from build123d import *

# Parameters (mm, degrees)
SKETCH1_R               = 19.53
BOSS_EXTRUDE1_DEPTH     = 1
BOSS_EXTRUDE3_START     = 1
SKETCH6_R               = 19.53
SKETCH6_R_2             = 9.525
BOSS_EXTRUDE3_DEPTH     = 1
THREAD1_PITCH           = 0.25
CUT_EXTRUDE1_DEPTH      = 28.691908616
CUT_EXTRUDE1_DEPTH_BACK = 28.691908616
SKETCH7_R               = 0.25
CUT_EXTRUDE2_DEPTH      = 28.691908616
CUT_EXTRUDE2_DEPTH_BACK = 28.691908616
SKETCH8_R               = 1


with BuildPart() as part:
    # Sketch1 → Boss-Extrude1 (new body)
    with BuildSketch(Plane(origin=(0, 0, 0), x_dir=(1, 0, 0), z_dir=(0, 1, 0))):
        with Locations(Location((0, 0, 0), (0, 0, 270))):
            Circle(SKETCH1_R)
    extrude(amount=BOSS_EXTRUDE1_DEPTH)

    # Sketch6 → Boss-Extrude3 (add)
    with BuildSketch(Plane.XZ.offset(BOSS_EXTRUDE3_START)):
        with Locations(Location((0, 0, 0), (0, 0, 270))):
            Circle(SKETCH6_R)
        with Locations(Location((0, 0, 0), (0, 0, 270))):
            Circle(SKETCH6_R_2, mode=Mode.SUBTRACT)
    extrude(amount=-BOSS_EXTRUDE3_DEPTH)

    # Thread1: the profile of Thread Profile1 profile screwed along a right-hand helix of 4 turns, 6 arcs to a turn; built about Z, then put on its axis
    thread1_z = Axis((0, 0, 0), (0, 0, 1))
    thread1_corners = [(9.5247, 0, -0.000173205), (9.660316469, 0, 0.078125), (9.660316469, 0, 0.109375), (9.5247, 0, 0.187673204)]
    with BuildLine(mode=Mode.PRIVATE) as thread1_profile:
        Line(thread1_corners[0], thread1_corners[1])
        Line(thread1_corners[1], thread1_corners[2])
        Line(thread1_corners[2], thread1_corners[3])
        Line(thread1_corners[3], thread1_corners[0])
    thread1_cap = Face(thread1_profile.wire())
    thread1_turn_angles = [0, 30, 60, 90, 120, 150, 180, 210, 240, 270, 300, 330, 360]
    thread1_turn_weights = [1, 0.8660254037844387, 1, 0.8660254037844387, 1, 0.8660254037844387, 1, 0.8660254037844387, 1, 0.8660254037844387, 1, 0.8660254037844387, 1]
    thread1_turn_rails = [Edge.make_bspline([Vector(p[0], p[1], 0).rotate(thread1_z, thread1_turn_angles[k]) / thread1_turn_weights[k] + Vector(0, 0, p[2] + THREAD1_PITCH * thread1_turn_angles[k] / 360) for k in range(13)], [0, 0, 0, 1, 1, 2, 2, 3, 3, 4, 4, 5, 5, 6, 6, 6], 2, thread1_turn_weights) for p in thread1_corners]
    thread1_turn_sides = [Face.make_surface_from_curves(thread1_turn_rails[p[0]], thread1_turn_rails[p[1]]) for p in [(0, 1), (1, 2), (2, 3), (3, 0)]]
    thread1 = Plane(origin=(0, -1, 0), x_dir=(1, 0, 0), z_dir=(0, 1, 0)) * Solid(Shell([*[p.moved(Location((0, 0, THREAD1_PITCH * i))) for i in range(4) for p in thread1_turn_sides], thread1_cap, thread1_cap.rotate(thread1_z, 1440).moved(Location((0, 0, THREAD1_PITCH * 1440 / 360)))]))
    add(thread1, mode=Mode.SUBTRACT)

    # Sketch7 → Cut-Extrude1 (cut, two sides: drawn at the far end of the back side and taken through both)
    with BuildSketch(Plane(origin=(0, 1, 0), x_dir=(1, 0, 0), z_dir=(0, 1, 0)).offset(-CUT_EXTRUDE1_DEPTH_BACK)):
        with Locations(Location((0, -10.25, 0), (0, 0, 270))):
            Circle(SKETCH7_R)
    extrude(amount=CUT_EXTRUDE1_DEPTH + CUT_EXTRUDE1_DEPTH_BACK, mode=Mode.SUBTRACT)

    # Sketch8 → Cut-Extrude2 (cut, two sides: drawn at the far end of the back side and taken through both)
    with BuildSketch(Plane(origin=(0, 1, 0), x_dir=(1, 0, 0), z_dir=(0, 1, 0)).offset(-CUT_EXTRUDE2_DEPTH_BACK)):
        with Locations(Location((7.778174593, 7.778174593, 0), (0, 0, 270))):
            Circle(SKETCH8_R)
    extrude(amount=CUT_EXTRUDE2_DEPTH + CUT_EXTRUDE2_DEPTH_BACK, mode=Mode.SUBTRACT)


solid = part.part
Verification items for the finished model (mm, model axes). Give positions to 0.01 mm unless a question says otherwise; leave off trailing zeros. Loops run counter-clockwise (first coordinate to the right, second up) from the corner with the lowest first, then second, coordinate; pieces in that order, holes last.
1) Draft check along Z on faces 1 (the flat face through (0, 0, 0)), 2 (the flat face through (0, 1, 0)). Enter one of: pulls with the +Z half, pulls with the -Z half, needs draft (parallel to the pull), parting line crosses it, or undercut.
2) Sectioned sample at C-C, the plane z = 12. Enter the section's corners in (x, y).
3) Depth check by flat-ended pin: pin 1 Ø17 at (x, z) = (0, 0) entering from -Y; pin 2 Ø22 at (x, z) = (0, 0) entering from -Y. Enter the tip coordinate at first touch or a pass-through.
4) Sectioned sample at B-B, the plane x = 17. Enter the section's corners in (y, z).
5) Sectioned sample at A-A, the plane y = 0.6. Enter the section's corners in (x, z), then the cut area to 3 significant figures.
6) Thickness scan on line 1 along Y through (x, z) = (3, -1); line 2 along X through (y, z) = (-0.5, 10.25); line 3 along X through (y, z) = (0.3, -2.5). Record the ranges inside material, lowest first.
Answers:
1. face 1: undercut
1. face 2: needs draft
2. outline: (-15.41, -1) - (15.41, -1) - (15.41, 1) - (-15.41, 1) - close
3. pin 1: stops at y = 0
3. pin 2: stops at y = -1
4. outline: (-1, -9.61) - (1, -9.61) - (1, 9.61) - (-1, 9.61) - close
5. outline: circle Ø39.06 at (0, 0); hole circle Ø0.5 at (0, 10.25); hole circle Ø2 at (7.78, -7.78)
5. area: 1,190 mm2
6. line 1: y = 0 to 1
6. line 2: x = -16.62 to -0.25, 0.25 to 16.62
6. line 3: x = -19.37 to 19.37
